from build123d import *

# Parameters (mm, degrees)
BOSS_EXTRUDE1_DEPTH = 5
SKETCH2_W           = 30
SKETCH2_H           = 70
CUT_EXTRUDE1_DEPTH  = 5
CUT_EXTRUDE2_DEPTH  = 5
SKETCH5_R           = 2.5
SKETCH5_R_2         = 5
CUT_EXTRUDE3_DEPTH  = 5
SKETCH6_R           = 2.5
CUT_EXTRUDE4_DEPTH  = 5
SKETCH7_R           = 12.5
SKETCH7_R_2         = 2.5
CUT_EXTRUDE5_DEPTH  = 5
SKETCH8_R           = 1.5
CUT_EXTRUDE6_DEPTH  = 5


with BuildPart() as part:
    # Sketch1 → Boss-Extrude1 (new body)
    with BuildSketch(Plane.XY):
        with BuildLine():
            Line((-90, -100), (90, -100))
            ThreePointArc((90, -100), (97.071067812, -97.071067812), (100, -90))
            Line((100, -90), (100, 70))
            ThreePointArc((100, 70), (91.213203436, 91.213203436), (70, 100))
            Line((70, 100), (-70, 100))
            ThreePointArc((-70, 100), (-91.213203436, 91.213203436), (-100, 70))
            Line((-100, 70), (-100, -90))
            ThreePointArc((-100, -90), (-97.071067812, -97.071067812), (-90, -100))
        make_face()
    extrude(amount=BOSS_EXTRUDE1_DEPTH)

    # Sketch2 → Cut-Extrude1 (cut)
    with BuildSketch(Plane.XY.offset(5)):
        with Locations((85, -55)):
            Rectangle(SKETCH2_W, SKETCH2_H)
        with Locations((-85, -55)):
            Rectangle(SKETCH2_W, SKETCH2_H)
    extrude(amount=-CUT_EXTRUDE1_DEPTH, mode=Mode.SUBTRACT)

    # Sketch3 → Cut-Extrude2 (cut)
    with BuildSketch(Plane.XY.offset(5)):
        with BuildLine():
            Line((85, -20), (100, -20))
            Line((100, -20), (100, 70))
            add(Edge.make_bspline(
                [(100, 70), (41.562750789, 76.769648156), (85, -20)],
                knots=[0, 0, 0, 1, 1, 1], degree=2))
        make_face()
        with BuildLine():
            Line((-85, -20), (-100, -20))
            Line((-100, -20), (-100, 70))
            add(Edge.make_bspline(
                [(-100, 70), (-41.562750789, 76.769648156), (-85, -20)],
                knots=[0, 0, 0, 1, 1, 1], degree=2))
        make_face()
    extrude(amount=-CUT_EXTRUDE2_DEPTH, mode=Mode.SUBTRACT)

    # Sketch5 → Cut-Extrude3 (cut)
    with BuildSketch(Plane.XY.offset(5)):
        with Locations((45, -80)):
            Circle(SKETCH5_R)
        with Locations((-45, -80)):
            Circle(SKETCH5_R)
        with Locations(Location((45, -20, 0), (0, 0, 180))):
            Circle(SKETCH5_R)
        with Locations(Location((-45, -20, 0), (0, 0, 180))):
            Circle(SKETCH5_R)
        with Locations((-45, 43.350998567)):
            Circle(SKETCH5_R_2)
        with Locations(Location((45, 43.350998567, 0), (0, 0, 180))):
            Circle(SKETCH5_R_2)
        with Locations((0, -30)):
            Circle(SKETCH5_R)
    extrude(amount=-CUT_EXTRUDE3_DEPTH, mode=Mode.SUBTRACT)

    # Sketch6 → Cut-Extrude4 (cut)
    with BuildSketch(Plane.XY.offset(5)):
        with Locations((0, -90)):
            Circle(SKETCH6_R)
    extrude(amount=-CUT_EXTRUDE4_DEPTH, mode=Mode.SUBTRACT)

    # Sketch7 → Cut-Extrude5 (cut)
    with BuildSketch(Plane(origin=(0, 0, 0), x_dir=(-1, 0, 0), z_dir=(0, 0, -1))):
        with Locations((0, 40)):
            Circle(SKETCH7_R)
        with Locations((-21, 40)):
            Circle(SKETCH7_R_2)
        with Locations((21.26, 40)):
            Circle(SKETCH7_R_2)
    extrude(amount=-CUT_EXTRUDE5_DEPTH, mode=Mode.SUBTRACT)

    # Sketch8 → Cut-Extrude6 (cut)
    with BuildSketch(Plane.XY.offset(5)):
        with Locations((-80, 80)):
            Circle(SKETCH8_R)
        with Locations((80, 80)):
            Circle(SKETCH8_R)
    extrude(amount=-CUT_EXTRUDE6_DEPTH, mode=Mode.SUBTRACT)


solid = part.part
Model file for the job. Use its own axes, mm. A direction names the side the tool comes from. Coordinates: 2 decimals unless noted, no trailing zeros. Loops run counter-clockwise (first coordinate to the right, second up) from the corner with the lowest first, then second, coordinate; pieces in that order, holes last. Notation, with made-up numbers: (-27.5, 88) -> (25.5, 88) arc R17 cw to (25.5, 109) -> close; hole circle Ø2 at (15.25, 13.5). An arc over 180 degrees is marked (long way). Use one line per item in the form item = value. Start each with the question number.
(1) Cut at D-D on y = -58. Give the cut face in (x, z), and give its area (3 significant figures).
(2) Cut at C-C on x = 45. Give the cut face in (y, z).
(3) Flat gauge pins, fed straight in: pin 1 (8 mm diameter, centred on x = -45, y = -80, fed in from +Z); pin 2 (1 mm diameter, centred on y = 75, z = 3, fed in from -X); pin 3 (2.5 mm diameter, centred on x = 82.5, z = 3, fed in from +Y); pin 4 (2.5 mm diameter, centred on y = -39, z = 2, fed in from +X). Where does each tip first touch, or does it go through?
(4) Pull direction X, two halves, no side cores. Call faces 4 (the cylindrical face through (-0.33, -87.52, 2.54)), 5 (the flat face through (-85, -90, 3)), 6 (the cylindrical face through (91.445, 90.979, 2.465)): pulls with the +X half, pulls with the -X half, needs draft (parallel to the pull), parting line crosses it, or undercut.
(5) Cut at A-A on x = 21. Give the cut face in (y, z), and give its area (3 significant figures).
(6) Probe probe 1 along Y at (x, z) = (-45, 4); probe 2 along X at (y, z) = (-79.5, 1.65); probe 3 along Y at (x, z) = (0.5, 2.9). List the from-to ranges inside material, lowest first. Write a range as from..to.
(7) Cut at B-B on y = -30. Give the cut face in (x, z).
(8) Tool access for faces 1 (the cylindrical face through (-97.15, -96.99, 2.46)), 2 (the flat face through (-78, -20, 3)), 3 (the flat face through (70, -55, 3)): list every direction of +Z, -Z, +X, -X, +Y, -Y with a clear straight run to the whole face (end or side of a thin tool).
Values:
q1.outline = (-70, 0) -> (70, 0) -> (70, 5) -> (-70, 5) -> close
q1.area = 700 mm2
q2.outline = (-100, 0) -> (-82.5, 0) -> (-82.5, 5) -> (-100, 5) -> close; (-77.5, 0) -> (-22.5, 0) -> (-22.5, 5) -> (-77.5, 5) -> close; (-17.5, 0) -> (38.35, 0) -> (38.35, 5) -> (-17.5, 5) -> close; (48.35, 0) -> (100, 0) -> (100, 5) -> (48.35, 5) -> close
q3.pin_1 = 5
q3.pin_2 = -99.66
q3.pin_3 = 97.81
q3.pin_4 = 70
q4.face_4 = undercut
q4.face_5 = needs draft
q4.face_6 = pulls with the +X half
q5.outline = (-100, 0) -> (37.5, 0) -> (37.5, 5) -> (-100, 5) -> close; (42.5, 0) -> (100, 0) -> (100, 5) -> (42.5, 5) -> close
q5.area = 975 mm2
q6.probe_1 = -100..-82.5, -77.5..-22.5, -17.5..38.35, 48.35..100
q6.probe_2 = -70..-47.45, -42.55..42.55, 47.45..70
q6.probe_3 = -100..-92.45, -87.55..-32.45, -27.55..27.51, 52.49..100
q7.outline = (-70, 0) -> (-2.5, 0) -> (-2.5, 5) -> (-70, 5) -> close; (2.5, 0) -> (70, 0) -> (70, 5) -> (2.5, 5) -> close
q8.face_1 = +Z, -Z, -X, -Y
q8.face_2 = +Z, -Z, -X
q8.face_3 = +Z, -Z, +X
